The model under review builds one solid part; all positions refer to its coordinate system, in mm. Face numbers are marked on the shaded views. Coordinates: 2 decimals unless noted, no trailing zeros. Loops run counter-clockwise (first coordinate to the right, second up) from the corner with the lowest first, then second, coordinate; pieces in that order, holes last. Notation, with made-up numbers: M 69.25,61.25 L 94.25,61.25 A7 cw 94.25,70.25 Z; hole C 45,33.5 d9. An arc over 180 degrees is marked long. One line per item, written item: value.
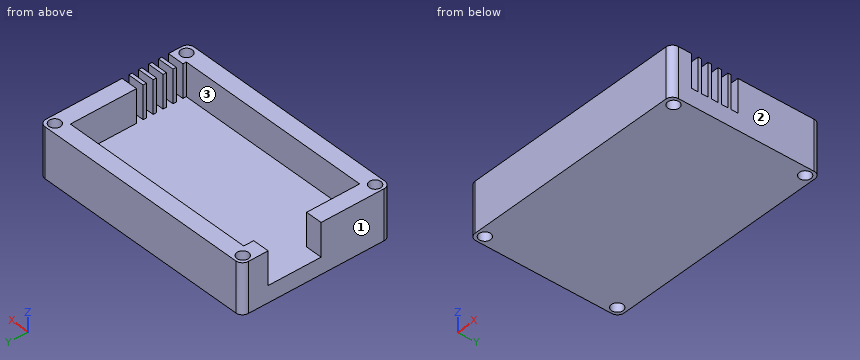
Autodesk Fusion 360 part; units mm, degrees
sketch "Sketch1" plane through (0, 0, 0) normal (0, 0, 1) x (1, 0, 0)
  line L0 (0, 0) -> (70, 0)
  line L1 (70, 0) -> (70, 45)
  line L2 (70, 45) -> (0, 45)
  line L3 (0, 45) -> (0, 0)
  line L4 (5, 40) -> (65, 40)
  line L5 (65, 40) -> (65, 5)
  line L6 (65, 5) -> (5, 5)
  line L7 (5, 5) -> (5, 40)
  line L8 (70, 19) -> (70, 21)
  line L9 (70, 16) -> (70, 18)
  line L10 (65, 18) -> (65, 16)
  line L11 (65, 15) -> (65, 13)
  line L12 (70, 10) -> (70, 12)
  line L13 (65, 12) -> (65, 10)
  line L14 (0, 37) -> (5, 37)
  line L15 (5, 37) -> (5, 21)
  line L16 (5, 21) -> (0, 21)
  line L17 (0, 21) -> (0, 37)
  line L18 (65, 18) -> (70, 18)
  line L19 (70, 18) -> (70, 20)
  line L20 (70, 20) -> (65, 20)
  line L21 (65, 20) -> (65, 18)
  line L22 (65, 15) -> (70, 15)
  line L23 (70, 15) -> (70, 17)
  line L24 (70, 17) -> (65, 17)
  line L25 (65, 17) -> (65, 15)
  line L26 (65, 12) -> (70, 12)
  line L27 (70, 12) -> (70, 14)
  line L28 (70, 14) -> (65, 14)
  line L29 (65, 14) -> (65, 12)
  line L30 (65, 11) -> (70, 11)
  line L31 (70, 11) -> (70, 9)
  line L32 (70, 9) -> (65, 9)
  line L33 (65, 9) -> (65, 11)
  line L34 (70, 8) -> (65, 8)
  line L35 (65, 8) -> (65, 6)
  line L36 (65, 6) -> (70, 6)
  line L37 (70, 6) -> (70, 8)
  circle A0 centre (67.5, 42.5) radius 1.75
  circle A1 centre (2.5, 2.5) radius 1.75
  circle A2 centre (2.5, 42.5) radius 1.75
  circle A3 centre (67.5, 2.7406) radius 1.75
  point P0 (-50.3404, 3.4837)
  dimension "d1" = 45
  dimension "d2" = 70
  dimension "d3" = 35
  dimension "d4" = 60
  dimension "d5" = 5
  dimension "d6" = 5
  dimension "d7" = 16
  dimension "d8" = 3.5
  dimension "d9" = 2.5
  dimension "d10" = 2.5
  dimension "d11" = 3.5
  dimension "d12" = 2.5
  dimension "d13" = 2.5
  dimension "d14" = 3.5
  dimension "d15" = 2.5
  dimension "d16" = 2.5
  dimension "d17" = 3.5
  dimension "d18" = 2.5
extrude "Extrude1" add sketch "Sketch1" along normal blind 15 contours L0 L1 L3 L5 L6 L7 L16 L36 | L1 L2 L3 L4 L5 L7 L8 L14 L20 | L1 L5 L32 L34 | L1 L5 L12 L13 L26 L30 | L1 L5 L9 L10 L18 L24 | L1 L5 L11 L22 L28 makes body 1 at (66.6667, 11, 5) makes body 2 at (46.6667, 45, 10) makes body 3 at (68.3333, 14, 5) makes body 4 at (68.3333, 9, 5) makes body 5 at (23.3333, 0, 10) makes body 6 at (66.6667, 18, 5)
extrude "Extrude2" add sketch "Sketch1" along normal blind 5 separate body contours L4 L5 L6 L7 L10 L11 L13 L15 L21 L25 L29 L33 L35 makes body 7
fillet "Fillet1" radius 2 4 edges at (70, 45, 7.5) (0, 45, 7.5) (70, 0, 7.5) (0, 0, 7.5) on bodies 2 5
extrude "Extrude3" add sketch "Sketch1" along normal blind 5 contours L3 L7 L14 L15 L16 L17 bodies 2 5 7
extrude "Extrude4" add sketch "Sketch1" along normal blind 5 contours L1 L5 L34 L35 L36 L37 | L1 L5 L12 L13 L30 L31 L32 L33 | L1 L5 L8 L18 L19 L20 L21 | L1 L5 L11 L26 L27 L28 L29 | L1 L5 L9 L10 L22 L23 L24 L25 bodies 1 2 3 4 6
(1) To check wall thickness, follow L1, parallel to Y at x = 2.5, z = 9; L2, parallel to Y at x = 32, z = 14.25; L3, parallel to X at y = 20.5, z = 9.5. State the ranges of each line that lie inside material, in increasing order. Write a range as [from, to].
Checks:
L1: [0, 0.75], [4.25, 21], [37, 40.75], [44.25, 45]
L2: [0, 5], [40, 45]
L3: [0, 5], [65, 70]
(2) Add section A-A on x = 53. State the section outline as (y, z) points, then the cut area to 3 significant figures.
Checks:
outline: M 0,0 L 45,0 L 45,15 L 40,15 L 40,5 L 5,5 L 5,15 L 0,15 Z
area: 325 mm^2
(3) Insertion check: pin 1 Ø5 at (x, y) = (14, 17.5) entering from +Z; pin 2 Ø3 at (y, z) = (33.5, 10) entering from -X. Each pin has a flat end and moves straight along its axis. Give the tip position at first contact, or say it passes through.
Checks:
pin 1: z = 5
pin 2: x = 65
(4) Add section B-B on z = 6.5. State how many separate pieces and enclosed holes the cut face has, then the cut area to 3 significant figures.
Checks:
separate pieces: 6
enclosed holes: 4
area: 878 mm^2
(5) Add section C-C on y = 30. State the section outline as (x, z) points, then the cut area to 3 significant figures.
Checks:
outline: M 0,0 L 70,0 L 70,15 L 65,15 L 65,5 L 0,5 Z
area: 400 mm^2
(6) Draft analysis for pull direction X (two halves, no side actions). For the marked faces 1, 2 and 3, state which applies: pulls with the +X half, pulls with the -X half, needs draft (parallel to the pull), parting line crosses it, or undercut.
Checks:
face 1: pulls with the -X half
face 2: pulls with the +X half
face 3: undercut
